Source: CAD feature listing. Evaluate the final solid. Frame: model axes, mm. A direction names the side the tool comes from. Round coordinates to 2 decimals unless told otherwise and drop trailing zeros. Loops run counter-clockwise (first coordinate to the right, second up) from the corner with the lowest first, then second, coordinate; pieces in that order, holes last. Notation, with made-up numbers: (15.5, 29.25) -> (51.5, 29.25) arc R16 cw to (51.5, 33.25) -> close; hole circle Ø11 at (-19.75, 64). An arc over 180 degrees is marked (long way). Write item = value, one per line.
from build123d import *

# Parameters (mm, degrees)
CUT_EXTRUDE1_DEPTH = 2.5
FILLET1_R          = 0.5
CHAMFER1_SIZE      = 0.25
CHAMFER2_SIZE      = 0.25


with BuildPart() as part:
    # Sketch1 → Revolve1 (revolve)
    with BuildSketch(Plane.XY):
        Polygon((0, 0), (4.25, 0), (4.25, -5), (2.5, -5), (2.5, -13), (0, -13), align=None)
    revolve(axis=Axis((0, -18, 0), (0, 1, 0)))

    # Sketch2 → Cut-Extrude1 (cut)
    with BuildSketch(Plane(origin=(0, 0, 0), x_dir=(1, 0, 0), z_dir=(0, 1, 0))):
        Polygon((2.309401077, 0), (1.154700538, 2), (-1.154700538, 2), (-2.309401077, 0), (-1.154700538, -2), (1.154700538, -2), align=None)
    extrude(amount=-CUT_EXTRUDE1_DEPTH, mode=Mode.SUBTRACT)

    # Fillet1
    fillet1_edges = [part.edges().sort_by_distance(p)[0] for p in [
        (-4.25, 0, 0),
    ]]
    fillet(fillet1_edges, radius=FILLET1_R)

    # Chamfer1
    chamfer1_edges = [part.edges().sort_by_distance(p)[0] for p in [
        (-4.25, -5, 0),
    ]]
    chamfer(chamfer1_edges, length=CHAMFER1_SIZE)

    # Chamfer2
    chamfer2_edges = [part.edges().sort_by_distance(p)[0] for p in [
        (-2.5, -13, 0),
    ]]
    chamfer(chamfer2_edges, length=CHAMFER2_SIZE)


solid = part.part
1. Set-up query: faces 1 (the face through (1.724, -1.232, 1.014)), 2 (the face through (0, -13, 0)). Return all of +Z, -Z, +X, -X, +Y, -Y with unobstructed straight access to the full face (end or side cutting, diameter ignored); none if empty.
Evaluation:
face_1 = +Y
face_2 = +Z, -Z, +X, -X, -Y
2. Contact query for flat-ended pins moving along their axis: pin 1 Ø3 at (x, z) = (-0.5, 0) entering from +Y; pin 2 Ø1 at (x, y) = (2.5, -2) entering from +Z; pin 3 Ø3 at (y, z) = (-8, 0) entering from +X. Output: stop coordinate, or through.
Evaluation:
pin_1 = -2.5
pin_2 = 3.75
pin_3 = 2.5
3. Section query B-B (x = 0). Return the cut outline in (y, z).
Evaluation:
outline = (-13, -2.25) -> (-12.75, -2.5) -> (-5, -2.5) -> (-5, -4) -> (-4.75, -4.25) -> (-0.5, -4.25) arc R0.5 ccw to (0, -3.75) -> (0, -2) -> (-2.5, -2) -> (-2.5, 2) -> (0, 2) -> (0, 3.75) arc R0.5 ccw to (-0.5, 4.25) -> (-4.75, 4.25) -> (-5, 4) -> (-5, 2.5) -> (-12.75, 2.5) -> (-13, 2.25) -> close
4. Section query A-A (y = -1). Return the cut outline in (x, z), then the cut area to 3 significant figures.
Evaluation:
outline = circle Ø8.5 at (0, 0); hole (-2.31, 0) -> (-1.15, -2) -> (1.15, -2) -> (2.31, 0) -> (1.15, 2) -> (-1.15, 2) -> close
area = 42.9 mm²
5. Line query: probe 1 along Y at (x, z) = (3, -1); probe 2 along Z at (x, y) = (-1.5, -8.75); probe 3 along X at (y, z) = (-10, 0). Output: solid intervals per line, ascending. Write a range as from..to.
Evaluation:
probe_1 = -5..0
probe_2 = -2..2
probe_3 = -2.5..2.5
6. Mould query, pull axis Z, two halves, no side actions, for faces 3 (the face through (2, -5, -2)), 4 (the face through (-0.54, -8.93, 2.44)), 5 (the face through (0, -2.5, 0)). Classes: released by +Z, released by -Z, zero draft, split by the parting line, or undercut.
Evaluation:
face_3 = zero draft
face_4 = split by the parting line
face_5 = undercut
7. Section query C-C (y = -6). Return the cut outline in (x, z), then the cut area to 3 significant figures.
Evaluation:
outline = circle Ø5 at (0, 0)
area = 19.6 mm²
8. Section query D-D (y = -2.75). Return the cut outline in (x, z).
Evaluation:
outline = circle Ø8.5 at (0, 0)
